Can you work these out from the model? Positions are in its coordinate system, mm. A direction names the side the tool comes from. Give positions to 0.01 mm unless a question says otherwise; leave off trailing zeros. Loops run counter-clockwise (first coordinate to the right, second up) from the corner with the lowest first, then second, coordinate; pieces in that order, holes last. Notation, with made-up numbers: (37, 9.25) -> (61, 9.25) arc R16 ccw to (61, 28.25) -> close; hole circle Ø10 at (22, -26.5). An arc over 180 degrees is marked (long way). Use CSV: the item, a comma, the result in double quotes.
from build123d import *

# Parameters (mm, degrees)
CROQUIS1_W              = 20
CROQUIS1_H              = 10
CROQUIS1_R              = 1.55
SALIENTE_EXTRUIR1_DEPTH = 3
CROQUIS2_W              = 3
CROQUIS2_H              = 10
SALIENTE_EXTRUIR2_DEPTH = 12
CROQUIS3_R              = 1.55
CORTAR_EXTRUIR1_DEPTH   = 3
CORTAR_EXTRUIR3_DEPTH   = 1
REDONDEO1_R             = 3
REDONDEO2_R             = 4
CORTAR_EXTRUIR4_DEPTH   = 1


with BuildPart() as part:
    # Croquis1 → Saliente-Extruir1 (new body)
    with BuildSketch(Plane(origin=(0, 0, 0), x_dir=(1, 0, 0), z_dir=(0, 1, 0))):
        with Locations((10, 5)):
            Rectangle(CROQUIS1_W, CROQUIS1_H)
        with Locations(Location((12.5, 5, 0), (0, 0, 270))):
            Circle(CROQUIS1_R, mode=Mode.SUBTRACT)
    extrude(amount=SALIENTE_EXTRUIR1_DEPTH)

    # Croquis2 → Saliente-Extruir2 (add)
    with BuildSketch(Plane(origin=(0, 3, 0), x_dir=(1, 0, 0), z_dir=(0, 1, 0))):
        with Locations((1.5, 5)):
            Rectangle(CROQUIS2_W, CROQUIS2_H)
    extrude(amount=SALIENTE_EXTRUIR2_DEPTH)

    # Croquis3 → Cortar-Extruir1 (cut)
    with BuildSketch(Plane.ZY):
        with Locations((-5, 9.5)):
            Circle(CROQUIS3_R)
    extrude(amount=-CORTAR_EXTRUIR1_DEPTH, mode=Mode.SUBTRACT)

    # Croquis5 → Cortar-Extruir3 (cut)
    with BuildSketch(Plane(origin=(3, 0, 0), x_dir=(0, 0, -1), z_dir=(1, 0, 0))):
        Polygon((7.9, 11.174315781), (5, 12.848631561), (2.1, 11.174315781), (2.1, 7.825684219), (5, 6.151368439), (7.9, 7.825684219), align=None)
    extrude(amount=-CORTAR_EXTRUIR3_DEPTH, mode=Mode.SUBTRACT)

    # Redondeo1
    redondeo1_edges = [part.edges().sort_by_distance(p)[0] for p in [
        (1.5, 15, 0),
        (1.5, 15, -10),
        (20, 1.5, -10),
        (20, 1.5, 0),
    ]]
    fillet(redondeo1_edges, radius=REDONDEO1_R)

    # Redondeo2
    # the kernel refuses this fillet: 4 mm, written as the material it adds along each edge
    with BuildSketch(Plane(origin=(3, 3, -10), x_dir=(0, 1, 0), z_dir=(0, 0, 1))) as redondeo2_piece_1_section:
        with BuildLine():
            CenterArc((REDONDEO2_R, -REDONDEO2_R), REDONDEO2_R, 90, 90)
            Line((0, -REDONDEO2_R), (0, 0))
            Line((0, 0), (REDONDEO2_R, 0))
        make_face()
    redondeo2_piece_1 = extrude(amount=10, mode=Mode.PRIVATE)
    redondeo2_piece_1 = split(redondeo2_piece_1, bisect_by=Plane(origin=(3.346509798, 4.243965629, -8.303718576), z_dir=(0, 0.8660254037844384, -0.5000000000000007)), keep=Keep.TOP, mode=Mode.PRIVATE)
    redondeo2_piece_1 = split(redondeo2_piece_1, bisect_by=Plane(origin=(3.346509798, 7.41640276, -7.191103718), z_dir=(0, -0.8660254037844387, -0.5)), keep=Keep.TOP, mode=Mode.PRIVATE)
    add(redondeo2_piece_1)
    with BuildSketch(Plane(origin=(3, 3, -10), x_dir=(0, 1, 0), z_dir=(0, 0, 1))) as redondeo2_piece_2_section:
        with BuildLine():
            CenterArc((REDONDEO2_R, -REDONDEO2_R), REDONDEO2_R, 90, 90)
            Line((0, -REDONDEO2_R), (0, 0))
            Line((0, 0), (REDONDEO2_R, 0))
        make_face()
    redondeo2_piece_2 = extrude(amount=10, mode=Mode.PRIVATE)
    redondeo2_piece_2 = split(redondeo2_piece_2, bisect_by=Plane(origin=(4.081067975, 5.513393982, -6.105004173), z_dir=(0, -0.8660254037844384, 0.5000000000000007)), keep=Keep.TOP, mode=Mode.PRIVATE)
    redondeo2_piece_2 = split(redondeo2_piece_2, bisect_by=Plane(origin=(4.081067975, 5.513393982, -3.894995827), z_dir=(0, -0.8660254037844387, -0.5)), keep=Keep.TOP, mode=Mode.PRIVATE)
    add(redondeo2_piece_2)
    with BuildSketch(Plane(origin=(3, 3, -10), x_dir=(0, 1, 0), z_dir=(0, 0, 1))) as redondeo2_piece_3_section:
        with BuildLine():
            CenterArc((REDONDEO2_R, -REDONDEO2_R), REDONDEO2_R, 90, 90)
            Line((0, -REDONDEO2_R), (0, 0))
            Line((0, 0), (REDONDEO2_R, 0))
        make_face()
    redondeo2_piece_3 = extrude(amount=10, mode=Mode.PRIVATE)
    redondeo2_piece_3 = split(redondeo2_piece_3, bisect_by=Plane(origin=(3.346509798, 7.41640276, -2.808896282), z_dir=(0, -0.8660254037844384, 0.5000000000000007)), keep=Keep.TOP, mode=Mode.PRIVATE)
    redondeo2_piece_3 = split(redondeo2_piece_3, bisect_by=Plane(origin=(3.346509798, 4.243965629, -1.696281424), z_dir=(0, 0.8660254037844387, 0.5)), keep=Keep.TOP, mode=Mode.PRIVATE)
    add(redondeo2_piece_3)

    # Croquis6 → Cortar-Extruir4 (cut)
    with BuildSketch(Plane(origin=(0, 3, 0), x_dir=(1, 0, 0), z_dir=(0, 1, 0))):
        Polygon((14.174315781, 7.9), (10.825684219, 7.9), (9.151368439, 5), (10.825684219, 2.1), (14.174315781, 2.1), (15.848631561, 5), align=None)
    extrude(amount=-CORTAR_EXTRUIR4_DEPTH, mode=Mode.SUBTRACT)


solid = part.part
(1) If we section it at A-A, the plane x = 12.5: Write out the boundary of the cut face in (y, z), then the cut area to 3 significant figures.
Answer sheet:
outline,"(0, -10) -> (3, -10) -> (3, -7.9) -> (2, -7.9) -> (2, -6.55) -> (0, -6.55) -> close; (0, -3.45) -> (2, -3.45) -> (2, -2.1) -> (3, -2.1) -> (3, 0) -> (0, 0) -> close"
area,"18.0 mm2"
(2) We'd pull the mould along Z, two halves only. Please class faces 1 (the face through (19.1, 1.52, -9.14)), 2 (the face through (5, 3, 0)), 3 (the face through (12.5, 2.5, -7.9)), 4 (the face through (1, 15, -5)): released by +Z, released by -Z, zero draft, split by the parting line, or undercut.
Answer sheet:
face 1,"released by -Z"
face 2,"released by +Z"
face 3,"undercut"
face 4,"zero draft"
(3) Will these pins go through, and if not, where does the flat tip stop? pin 1 Ø6 at (x, z) = (16, -5) entering from -Y; pin 2 Ø6 at (y, z) = (11, -8.5) entering from +X; pin 3 Ø4.5 at (x, z) = (12.5, -4) entering from +Y; pin 4 Ø1 at (y, z) = (7, -5) entering from +X.
Answer sheet:
pin 1,"stops at y = 0"
pin 2,"stops at x = 3"
pin 3,"stops at y = 3"
pin 4,"stops at x = 2"
(4) If we section it at C-C, the plane x = 1.5: Write out the boundary of the cut face in (y, z), then the cut area to 3 significant figures.
Answer sheet:
outline,"(0, -10) -> (12, -10) arc R3 ccw to (15, -7) -> (15, -3) arc R3 ccw to (12, 0) -> (0, 0) -> close; hole circle Ø3.1 at (9.5, -5)"
area,"139 mm2"
(5) If I drill on L1, parallel to Z at x = 12.5, y = 0.6; L2, parallel to X at y = 1.45, z = -5; L3, parallel to Y at x = 0.5, z = -5, over which ranges is the centre line in solid material (lowest first)? Write a range as from..to.
Answer sheet:
L1,"z = -10..-6.55, -3.45..0"
L2,"x = 0..10.95, 14.05..20"
L3,"y = 0..7.95, 11.05..15"
(6) Which directions (+Z, -Z, +X, -X, +Y, -Y) give clear straight access to the entire face, cutting with the end or side of a thin tool? Please do faces 5 (the face through (15.023, 2.507, -6.43)), 6 (the face through (2.507, 12.023, -3.57)), 7 (the face through (3, 13, -4)).
Answer sheet:
face 5,"+Y"
face 6,"+X"
face 7,"+Z, -Z, +X, +Y"
(7) If we section it at D-D, the plane z = -4.25: Write out the boundary of the cut face in (x, y), then the cut area to 3 significant figures.
Answer sheet:
outline,"(0, 0) -> (11.14, 0) -> (11.14, 2) -> (9.58, 2) -> (9.58, 3) -> (7, 3) arc R4 cw to (3.02, 6.58) -> (2, 6.58) -> (2, 8.14) -> (0, 8.14) -> close; (0, 10.86) -> (2, 10.86) -> (2, 12.42) -> (3, 12.42) -> (3, 15) -> (0, 15) -> close; (13.86, 0) -> (20, 0) -> (20, 3) -> (15.42, 3) -> (15.42, 2) -> (13.86, 2) -> close"
area,"76.9 mm2"
